Can you work these out from the drawing? Everything is in mm from the part's minimum corner. A direction names the side the tool comes from. Round coordinates to 2 decimals unless told otherwise and drop trailing zeros. Order: outer loops, then holes, each group sorted by start corner. A loop starts at its lowest first (then second) coordinate and runs counter-clockwise, first axis right, second up. Notation, with made-up numbers: (4, 63) -> (38, 63) arc R12 ccw to (38, 72) -> close; hole circle Ø3 at (-17, 11). An arc over 180 degrees is marked (long way). One line per item, written item: value.
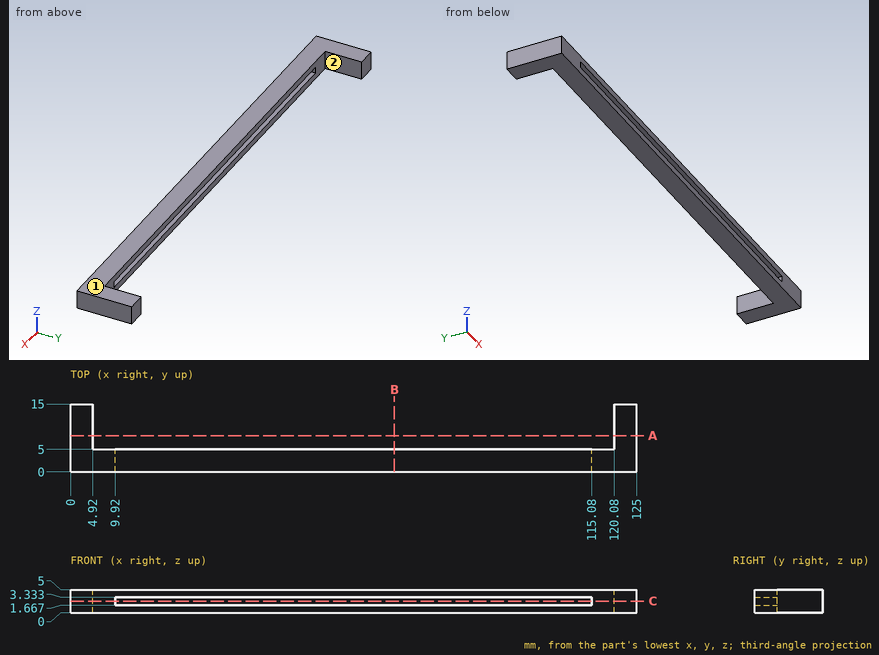
Q1. Which directions (+Z, -Z, +X, -X, +Y, -Y) give clear straight access to the entire face, cutting with the end or side of a thin tool? Please do the marked faces 1 and 2.
Answers:
face 1: +Z, +X, -X, +Y, -Y
face 2: +Z, -Z, +Y
Q2. I want a section at A-A on y = 8. Write out the boundary of the cut face in (x, z), then the cut area to 3 significant figures.
Answers:
outline: (0, 0) -> (4.92, 0) -> (4.92, 5) -> (0, 5) -> close; (120.08, 0) -> (125, 0) -> (125, 5) -> (120.08, 5) -> close
area: 49.2 mm2
Q3. For P1, Ø2.5, axis at x = 52.5, z = 1.5, coming from the +Y side; P2, Ø8, axis at x = 62.5, y = 12.5, coming from the -Z side, each with a flat end and sliding along its axis, tell me the tip position at first contact or that it passes through.
Answers:
P1: y = 5
P2: through
Q4. I want a section at B-B on x = 71.5. Write out the boundary of the cut face in (y, z).
Answers:
outline: (0, 0) -> (5, 0) -> (5, 1.67) -> (0, 1.67) -> close; (0, 3.33) -> (5, 3.33) -> (5, 5) -> (0, 5) -> close
Q5. I need wall thicknesses on line 1 along X through (y, z) = (13.25, 1.9); line 2 along X through (y, z) = (2.75, 2.8); line 3 along Z through (x, y) = (31, 1). Which ranges of each line are inside material? Lowest first, please.
Answers:
line 1: 0 to 4.92, 120.08 to 125
line 2: 0 to 9.92, 115.08 to 125
line 3: 0 to 1.67, 3.33 to 5
Q6. I want a section at C-C on z = 2.55. Write out the boundary of the cut face in (x, y), then the cut area to 3 significant figures.
Answers:
outline: (0, 0) -> (9.92, 0) -> (9.92, 5) -> (4.92, 5) -> (4.92, 15) -> (0, 15) -> close; (115.08, 0) -> (125, 0) -> (125, 15) -> (120.08, 15) -> (120.08, 5) -> (115.08, 5) -> close
area: 198 mm2
